from build123d import *

# Parameters (mm, degrees)
F1_ANGLE = 180
F6_R     = 3.175
F7_DEPTH = 71.401


with BuildPart() as f1:
    # F0 (on Front) → F1 (revolve)
    with BuildSketch(Plane.XZ):
        with BuildLine():
            ThreePointArc((43, 0), (39.7049512883, -7.9549512883), (31.75, -11.25))
            Line((31.75, -11.25), (0, -11.25))
            Line((0, -11.25), (-31.75, -11.25))
            Line((-31.75, -11.25), (-31.75, -14.25))
            Line((-31.75, -14.25), (31.75, -14.25))
            ThreePointArc((31.75, -14.25), (41.8262716319, -10.0762716319), (46, 0))
            Line((46, 0), (43, 0))
        make_face()
    revolve(axis=Axis((28.0016548932, 0, 0), (1, 0, 0)), revolution_arc=F1_ANGLE)

    # F4 (on face) → F5 (join, up to the next surface of F1)
    with BuildSketch(Plane(origin=(0, 26.95, 0), x_dir=(-1, 0, 0), z_dir=(0, 1, 0))):
        Polygon((25.4, 9.525), (6.35, 9.525), (6.35, 0), (6.35, -9.525), (25.4, -9.525), (25.4, 0), align=None)
        Polygon((-9.525, 0), (-9.525, 9.525), (-28.575, 9.525), (-28.575, 0), (-28.575, -9.525), (-9.525, -9.525), align=None)
    extrude(until=Until.NEXT, dir=(0, -1, 0))

    # F6 (on face) → F7 (cut, through all)
    with BuildSketch(Plane(origin=(-25.4, 0, 0), x_dir=(0, -1, 0), z_dir=(-1, 0, 0))):
        with Locations((-20.6, 0)):
            Circle(F6_R)
    extrude(amount=-F7_DEPTH, mode=Mode.SUBTRACT)


solid = f1.part
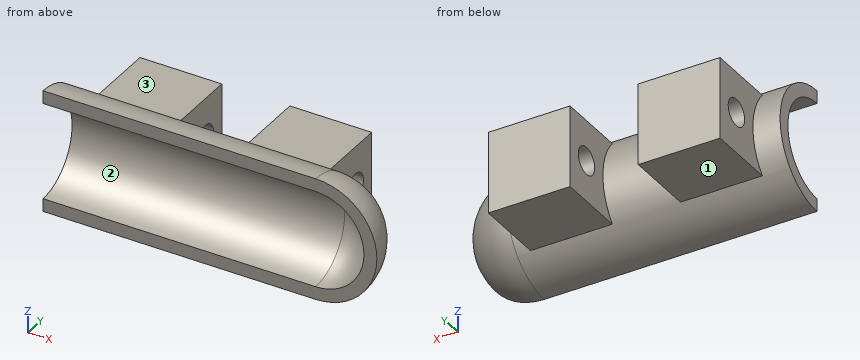
Geometry check sheet. Reference: the model listing, model coordinates, mm. Face numbers are marked on the shaded views. A direction names the side the tool comes from. Round coordinates to 2 decimals unless told otherwise and drop trailing zeros. Write each loop counter-clockwise with the first axis right and the second up, starting at its lowest first coordinate (ties: lowest second). Pieces come first, ordered by that corner, then holes. Notation, with made-up numbers: (16.5, -2) -> (28.5, -2) arc R23 cw to (28.5, 24) -> close; hole circle Ø8 at (29, 69.25). An arc over 180 degrees is marked (long way). One line per item, written item: value. Start each with the question number.
(1) Scan lines: line 1 (Z direction, x = 14.5, y = 20.6) (3 decimals); line 2 (X direction, y = 24, z = 6.25) (3 decimals); line 3 (Z direction, x = -14, y = 18.5) (3 decimals). Record each from-to range of solid material in increasing order. Write a range as [from, to].
(2) Cross-section at D-D, the plane y = 4.25. Record the cut outline in (x, z).
(3) Cross-section at A-A, the plane x = -15.5. Record the cut outline in (y, z) (3 decimals), and give its area (3 significant figures).
(4) Cross-section at C-C, the plane z = 0. Record the cut outline in (x, y) (3 decimals).
(5) Cross-section at B-B, the plane y = 20.6. Record the cut outline in (x, z) (3 decimals), and give its area (3 significant figures).
(6) Go/stop test with flat-tipped pins: pin 1 Ø5 at (x, y) = (-18.5, 20.5) entering from +Z (3 decimals); pin 2 Ø5 at (y, z) = (18.5, 11) entering from -X; pin 3 Ø8 at (y, z) = (19.5, 3) entering from +X (3 decimals). Record where each tip stops, or that it passes through.
(7) Access from +Z, -Z, +X, -X, +Y, -Y to the whole of each face (thin tool, end or side, straight path). Record for the marked faces 1, 2 and 3.
Answer:
1. line 1: [-9.525, -3.175], [3.175, 9.525]
1. line 2: [-25.4, -6.35], [9.525, 28.575]
1. line 3: [-9.525, -2.381], [2.381, 9.525]
2. outline: (-31.75, -13.6) -> (31.75, -13.6) arc R13.6 ccw to (31.75, 13.6) -> (-31.75, 13.6) -> (-31.75, 10.42) -> (31.75, 10.42) arc R10.42 cw to (31.75, -10.42) -> (-31.75, -10.42) -> close
3. outline: (0, -14.25) arc R14.25 ccw to (10.599, -9.525) -> (26.95, -9.525) -> (26.95, 9.525) -> (10.599, 9.525) arc R14.25 ccw to (0, 14.25) -> (0, 11.25) arc R11.25 cw to (0, -11.25) -> close; hole circle Ø6.35 at (20.6, 0)
3. area: 352 mm²
4. outline: (-31.75, 11.25) -> (31.75, 11.25) arc R11.25 cw to (43, 0) -> (46, 0) arc R14.25 ccw to (31.75, 14.25) -> (28.575, 14.25) -> (28.575, 17.425) -> (9.525, 17.425) -> (9.525, 14.25) -> (-6.35, 14.25) -> (-6.35, 17.425) -> (-25.4, 17.425) -> (-25.4, 14.25) -> (-31.75, 14.25) -> close; (-25.4, 23.775) -> (-6.35, 23.775) -> (-6.35, 26.95) -> (-25.4, 26.95) -> close; (9.525, 23.775) -> (28.575, 23.775) -> (28.575, 26.95) -> (9.525, 26.95) -> close
5. outline: (-25.4, -9.525) -> (-6.35, -9.525) -> (-6.35, -3.175) -> (-25.4, -3.175) -> close; (-25.4, 3.175) -> (-6.35, 3.175) -> (-6.35, 9.525) -> (-25.4, 9.525) -> close; (9.525, -9.525) -> (28.575, -9.525) -> (28.575, -3.175) -> (9.525, -3.175) -> close; (9.525, 3.175) -> (28.575, 3.175) -> (28.575, 9.525) -> (9.525, 9.525) -> close
5. area: 484 mm²
6. pin 1: z = 9.525
6. pin 2: x = -25.4
6. pin 3: x = 28.575
7. face 1: -Z, +X, -X, +Y
7. face 2: -X, -Y
7. face 3: +Z, +X, -X, +Y
